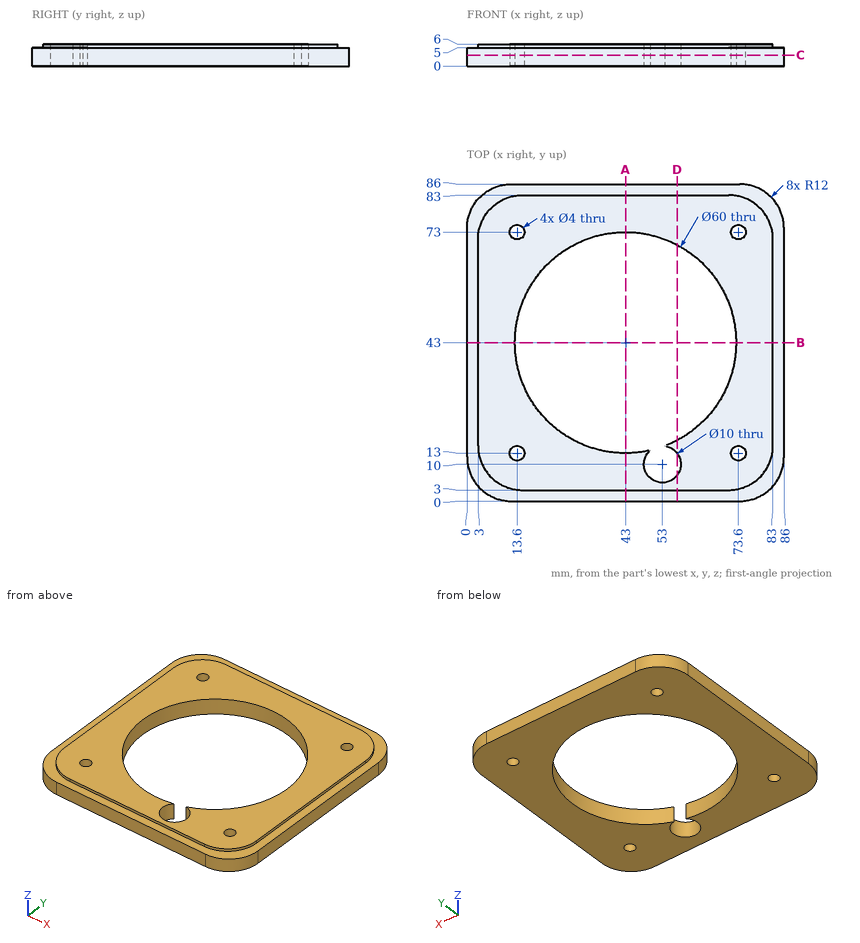
Part print with two shaded views. Sizes in mm from the minimum x, y, z corner. Round coordinates to 2 decimals unless told otherwise and drop trailing zeros. Order: outer loops, then holes, each group sorted by start corner. A loop starts at its lowest first (then second) coordinate and runs counter-clockwise, first axis right, second up. Notation, with made-up numbers: (65, -36) - (76, -36) arc R27 cw to (76, -7) - close; hole circle Ø11 at (25, -23.5). An arc over 180 degrees is marked (long way). Answer in a Markdown table with one row per item. Add a question column.
(1) Band-saw the part on D-D on x = 57. List the corners of the cut face in (y, z), and give its area (3 significant figures).
(2) Band-saw the part on C-C on z = 3. List the corners of the cut face in (x, y), and give its area (3 significant figures).
(3) Probe L1, parallel to Y at x = 73.6, z = 2.85; L2, parallel to X at y = 43.5, z = 5.65; L3, parallel to Y at x = 43, z = 3.3. List the from-to ranges inside material, lowest first. Write a range as [from, to].
(4) Drop flat-ended pins along their axis: pin 1 Ø3.5 at (x, y) = (73.6, 73) entering from -Z; pin 2 Ø1.1 at (y, z) = (41.5, 5.5) entering from -X; pin 3 Ø0.8 at (x, z) = (42.5, 5.5) entering from -Y; pin 4 Ø0.5 at (x, z) = (53.5, 5.5) entering from +Y. Give the stop position or say it passes through.
(5) Band-saw the part on A-A on x = 43. List the corners of the cut face in (y, z).
Data:
| question | item | result |
|---|---|---|
| 1 | outline | (0, 0) - (7, 0) - (7, 6) - (3, 6) - (3, 5) - (0, 5) - close; (13, 0) - (16.47, 0) - (16.47, 6) - (13, 6) - close; (69.53, 0) - (86, 0) - (86, 5) - (83, 5) - (83, 6) - (69.53, 6) - close |
| 1 | area | 156 mm^2 |
| 2 | outline | (0, 12) arc R12 ccw to (12, 0) - (74, 0) arc R12 ccw to (86, 12) - (86, 74) arc R12 ccw to (74, 86) - (12, 86) arc R12 ccw to (0, 74) - close; hole circle Ø4 at (13.6, 13); hole circle Ø4 at (13.6, 73); hole (49.7, 13.76) arc R5 ccw (long way) to (53.66, 14.96) arc R30 ccw (long way) to start; hole circle Ø4 at (73.6, 13); hole circle Ø4 at (73.6, 73) |
| 2 | area | 4,320 mm^2 |
| 3 | L1 | y = [0, 11], [15, 71], [75, 86] |
| 3 | L2 | x = [3, 13], [73, 83] |
| 3 | L3 | y = [0, 13], [73, 86] |
| 4 | pin 1 | passes through |
| 4 | pin 2 | stops at x = 0 |
| 4 | pin 3 | stops at y = 3 |
| 4 | pin 4 | stops at y = 83 |
| 5 | outline | (0, 0) - (13, 0) - (13, 6) - (3, 6) - (3, 5) - (0, 5) - close; (73, 0) - (86, 0) - (86, 5) - (83, 5) - (83, 6) - (73, 6) - close |
